```python
from build123d import *

# Parameters (mm, degrees)
SKETCH1_R                                            = 3.25
BOSS_EXTRUDE1_DEPTH                                  = 3
SKETCH7_R                                            = 1.25
CUT_EXTRUDE1_DEPTH                                   = 3
CSK_FOR_M3_HEX_SOCKET_COUNTERSUNK_HEAD_S_D           = 3.4
CSK_FOR_M3_HEX_SOCKET_COUNTERSUNK_HEAD_S_DEPTH       = 3
CSK_FOR_M3_HEX_SOCKET_COUNTERSUNK_HEAD_S_CSINK_D     = 6.94
CSK_FOR_M3_HEX_SOCKET_COUNTERSUNK_HEAD_S_CSINK_ANGLE = 90
CSK_FOR_M3_HEX_SOCKET_COUNTERSUNK_HEAD_S_TIP         = 1.021463052


with BuildPart() as part:
    # Sketch1 → Boss-Extrude1 (new body)
    with BuildSketch(Plane(origin=(14.780047825, 0, -21.146325355), x_dir=(-0.8196392423560167, 0, -0.5728800157014161), z_dir=(0.5728800157014161, 0, -0.8196392423560169))):
        with BuildLine():
            Line((13.893407272, 266.511550752), (18.893407272, 266.511550752))
            ThreePointArc((18.893407272, 266.511550752), (21.014727616, 265.632871095), (21.893407272, 263.511550752))
            Line((21.893407272, 263.511550752), (21.893407272, 255.611550752))
            ThreePointArc((21.893407272, 255.611550752), (21.014727616, 253.490230408), (18.893407272, 252.611550752))
            Line((18.893407272, 252.611550752), (3.879256414, 252.611550752))
            Line((3.879256414, 252.611550752), (3.879256414, 226.011550752))
            Line((3.879256414, 226.011550752), (12.21108842, 226.011550752))
            ThreePointArc((12.21108842, 226.011550752), (17.804454002, 228.802722193), (23.397819584, 226.011550752))
            Line((23.397819584, 226.011550752), (66.393407272, 226.011550752))
            Line((66.393407272, 226.011550752), (66.393407272, 286.011550752))
            Line((66.393407272, 286.011550752), (13.893407272, 286.011550752))
            Line((13.893407272, 286.011550752), (13.893407272, 266.511550752))
        make_face()
        with Locations((27.893407272, 249.061550752)):
            Circle(SKETCH1_R, mode=Mode.SUBTRACT)
        with Locations((41.893407272, 249.061550752)):
            Circle(SKETCH1_R, mode=Mode.SUBTRACT)
    extrude(amount=BOSS_EXTRUDE1_DEPTH)

    # Sketch7 → Cut-Extrude1 (cut)
    with BuildSketch(Plane(origin=(16.498687872, 0, -23.605243082), x_dir=(-0.8196392423560169, 0, -0.572880015701416), z_dir=(0.572880015701416, 0, -0.8196392423560169))):
        with Locations((28.393407272, 278.011550752)):
            Circle(SKETCH7_R)
        with Locations((51.393407272, 278.011550752)):
            Circle(SKETCH7_R)
        with Locations((28.393407272, 256.011550752)):
            Circle(SKETCH7_R)
        with Locations((51.393407272, 256.011550752)):
            Circle(SKETCH7_R)
    extrude(amount=-CUT_EXTRUDE1_DEPTH, mode=Mode.SUBTRACT)

    # CSK for M3 Hex Socket Countersunk Head Screw2
    with Locations(Plane(origin=(16.498687872, 0, -23.605243082), x_dir=(-0.8196392423560169, 0, -0.572880015701416), z_dir=(0.572880015701416, 0, -0.819639242356017))):
        with Locations((17.893407272, 276.261550752), (7.879256414, 239.311550752), (62.393407272, 230.011550752)):
            CounterSinkHole(CSK_FOR_M3_HEX_SOCKET_COUNTERSUNK_HEAD_S_D / 2, CSK_FOR_M3_HEX_SOCKET_COUNTERSUNK_HEAD_S_CSINK_D / 2, depth=CSK_FOR_M3_HEX_SOCKET_COUNTERSUNK_HEAD_S_DEPTH, counter_sink_angle=CSK_FOR_M3_HEX_SOCKET_COUNTERSUNK_HEAD_S_CSINK_ANGLE)
            with Locations((0, 0, -(CSK_FOR_M3_HEX_SOCKET_COUNTERSUNK_HEAD_S_DEPTH + CSK_FOR_M3_HEX_SOCKET_COUNTERSUNK_HEAD_S_TIP / 2))):  # 118° drill point
                Cone(0, CSK_FOR_M3_HEX_SOCKET_COUNTERSUNK_HEAD_S_D / 2, CSK_FOR_M3_HEX_SOCKET_COUNTERSUNK_HEAD_S_TIP, mode=Mode.SUBTRACT)


solid = part.part
```
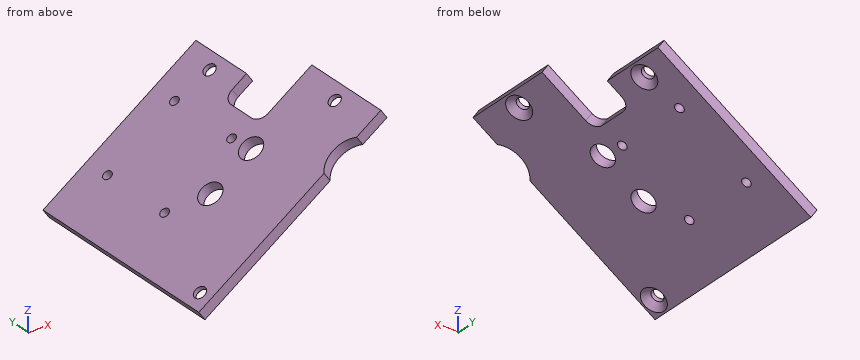
Source: CAD feature listing. Evaluate the final solid. Frame: model axes, mm. Give positions to 0.01 mm unless a question says otherwise; leave off trailing zeros. Order: outer loops, then holes, each group sorted by start corner. A loop starts at its lowest first (then second) coordinate and runs counter-clockwise, first axis right, second up.
(1) Contact query for flat-ended pins moving along their axis: P1, Ø1.5, axis at x = -32, y = 278.5, coming from the -Z side; P2, Ø10, axis at x = -30.5, y = 240, coming from the +Z side; P3, Ø5, axis at y = 275, z = -30.5, coming from the +X side. Output: stop coordinate, or through.
(2) Section query B-B (y = 267.5). Return the cut outline in (x, z).
(3) Material intervals for line 1 along X through (y, z) = (278, -43); line 2 along Z through (x, y) = (-26, 272.5); line 3 along X through (y, z) = (246, -40.5), sorted ascending.
(4) Section query A-A (y = 250). Return the cut outline in (x, z), plus the area to 3 significant figures.
Outcome:
1. P1: stops at z = -58.03
1. P2: stops at z = -49.3
1. P3: stops at x = 5.11
2. outline: (-39.64, -59.18) - (-37.92, -61.64) - (5.11, -31.56) - (3.39, -29.11) - close
3. line 1: x = -16.49 to -11.25
3. line 2: z = -53.31 to -49.65
3. line 3: x = -12.91 to -7.67
4. outline: (-39.64, -59.18) - (-37.92, -61.64) - (-20.39, -49.39) - (-22.11, -46.93) - close; (-17.01, -43.36) - (-15.29, -45.82) - (-8.91, -41.37) - (-10.63, -38.91) - close; (-5.53, -35.34) - (-3.81, -37.8) - (13.32, -25.83) - (11.6, -23.37) - close
4. area: 150 mm2
